Read the model definition and answer for the solid it produces. Units are mm, in the model's axes. A direction names the side the tool comes from. Coordinates: 2 decimals unless noted, no trailing zeros. Write each loop counter-clockwise with the first axis right and the second up, starting at its lowest first coordinate (ties: lowest second). Pieces come first, ordered by that corner, then holes. Notation, with made-up numbers: (82, 16) - (100, 16) arc R19 cw to (100, 40) - close; hole circle Ø5 at (85.5, 5). An arc over 180 degrees is marked (long way). Return JSON: item names as keys, results as strings.
Autodesk Inventor part; units mm, degrees
ref_plane "YZ Plane" through (0, 0, 0) normal (1, 0, 0) x (0, 1, 0)
ref_plane "XZ Plane" through (0, 0, 0) normal (0, 1, 0) x (-1, 0, 0)
ref_plane "XY Plane" through (0, 0, 0) normal (0, 0, 1) x (1, 0, 0)
sketch "Sketch1" plane through (0, 0, 0) normal (0, 1, 0) x (-1, 0, 0)
  line L0 (163.7334, -183.5335) -> (68.4834, -183.5335)
  line L1 (166.9084, -186.7085) -> (166.9084, -253.3835)
  line L2 (65.3084, -186.7085) -> (65.3084, -253.3835)
  arc A0 (166.9084, -186.7085) -> (163.7334, -183.5335) centre (163.7334, -186.7085) ccw
  arc A1 (68.4834, -183.5335) -> (65.3084, -186.7085) centre (68.4834, -186.7085) ccw
  line L3 (163.7334, -323.2335) -> (68.4834, -323.2335)
  line L4 (166.9084, -320.0585) -> (166.9084, -253.3835)
  line L5 (65.3084, -320.0585) -> (65.3084, -253.3835)
  arc A2 (163.7334, -323.2335) -> (166.9084, -320.0585) centre (163.7334, -320.0585) ccw
  arc A3 (65.3084, -320.0585) -> (68.4834, -323.2335) centre (68.4834, -320.0585) ccw
  point P0 (0, 0)
  point P1 (65.3084, -183.5335)
  dimension "d5" = 69.85
  dimension "d6" = 3.175
extrude "Extrusion1" add sketch "Sketch1" along normal blind 5.08
sketch "Sketch2" plane through (0, 5.08, 0) normal (0, 1, 0) x (1, 0, 0)
  arc A0 (-166.9084, 186.7085) -> (-163.7334, 183.5335) centre (-163.7334, 186.7085) ccw
  circle A1 centre (-163.7334, 186.7085) radius 1.27
  arc A2 (-68.4834, 183.5335) -> (-65.3084, 186.7085) centre (-68.4834, 186.7085) ccw
  circle A3 centre (-68.4834, 186.7085) radius 1.27
  arc A4 (-163.7334, 323.2335) -> (-166.9084, 320.0585) centre (-163.7334, 320.0585) ccw
  circle A5 centre (-163.7334, 320.0585) radius 1.27
  arc A6 (-65.3084, 320.0585) -> (-68.4834, 323.2335) centre (-68.4834, 320.0585) ccw
  circle A7 centre (-68.4834, 320.0585) radius 1.27
  point P0 (0, 0)
  dimension "d11" = 2.54
  dimension "d12" = 2.54
  dimension "d13" = 2.54
  dimension "d14" = 2.54
extrude "Extrusion2" cut sketch "Sketch2" against normal mid plane 25.4
sketch "Sketch3" plane through (0, 5.08, 0) normal (0, 1, 0) x (1, 0, 0)
  line L0 (-68.4834, 323.2335) -> (-163.7334, 323.2335)
  line L1 (-116.1084, 316.8835) -> (-80.3833, 316.8835)
  line L2 (-116.1084, 316.8835) -> (-151.8335, 316.8835)
  line L3 (-80.3833, 316.8835) -> (-80.3833, 310.5335)
  line L4 (-80.3833, 310.5335) -> (-151.8335, 310.5335)
  line L5 (-151.8335, 310.5335) -> (-151.8335, 316.8835)
  line L6 (-65.3084, 186.7085) -> (-65.3084, 320.0585)
  line L7 (-116.1084, 189.8835) -> (-80.3833, 189.8835)
  line L8 (-116.1084, 189.8835) -> (-151.8335, 189.8835)
  line L9 (-80.3833, 189.8835) -> (-80.3833, 196.2335)
  line L10 (-80.3833, 196.2335) -> (-151.8335, 196.2335)
  line L11 (-151.8335, 196.2335) -> (-151.8335, 189.8835)
  point P0 (0, 0)
extrude "Extrusion3" cut sketch "Sketch3" against normal blind 1.016
properties part number "Base Bracket 1x"
(1) A straight line is drawn through the part: line 1 (Z direction, x = -121, y = 4.85). Find the intervals that lie inside material, in ascending order. Write a range as from..to.
Answer:
{"line 1": "-323.23..-316.88, -310.53..-196.23, -189.88..-183.53"}
(2) Flat-ended cylindrical pins translate along their axes: P1, Ø2, axis at x = -163.73, z = -320.06, coming from the -Y side; P2, Ø1.9, axis at x = -123, z = -312.5, coming from the +Y side. Find the tip coordinate at first contact, or state that the pin passes through.
Answer:
{"P1": "through", "P2": "y = 4.06"}
(3) A cutting plane is placed at A-A (x = -107.5). Determine the outline of the cut face in (y, z), and give its area (3 significant figures).
Answer:
{"outline": "(0, -323.23) - (5.08, -323.23) - (5.08, -316.88) - (4.06, -316.88) - (4.06, -310.53) - (5.08, -310.53) - (5.08, -196.23) - (4.06, -196.23) - (4.06, -189.88) - (5.08, -189.88) - (5.08, -183.53) - (0, -183.53) - close", "area": "697 mm²"}
(4) Which of the six approach directions +Z, -Z, +X, -X, +Y, -Y give full straight-line access (tool end or side, diameter ignored) to faces 4 (the face through (-117, 4.064, -193)), 5 (the face through (-66.263, 2.504, -322.328))?
Answer:
{"face 4": "+Y", "face 5": "-Z, +X, +Y, -Y"}
(5) Determine the mould class of faces 1 (the face through (-115, 0, -252)), 2 (the face through (-117, 4.064, -314)), 3 (the face through (-117, 3, -183.534)) for opening direction Z: +Z half, -Z half, draft (parallel to the pull), parting line (faces both ways), or undercut.
Answer:
{"face 1": "draft", "face 2": "undercut", "face 3": "+Z half"}
